Autodesk Inventor part; units mm, degrees
ref_plane "YZ Plane" through (0, 0, 0) normal (1, 0, 0) x (0, 1, 0)
ref_plane "XZ Plane" through (0, 0, 0) normal (0, 1, 0) x (-1, 0, 0)
ref_plane "XY Plane" through (0, 0, 0) normal (0, 0, 1) x (1, 0, 0)
sketch "Sketch1" plane through (0, 0, 0) normal (1, 0, 0) x (0, 1, 0)
  circle A0 centre (0, 0) radius 20
  line L0 (8.5, 8.5) -> (-16.9, 8.5)
  line L1 (8.5, 8.5) -> (8.5, -16.9)
  line L2 (0, 0) -> (0, 20)
  line L3 (0, 20) -> (-60.9241, 20)
  line L4 (-60.9241, 20) -> (-60.9241, 18.5)
  line L5 (-60.9241, 18.5) -> (0, 18.5)
  line L6 (0, 18.5) -> (0, 20)
  line L7 (0, 0) -> (14.1421, 14.1421)
  line L8 (0, 0) -> (20, 0)
  line L9 (-16.9, 8.5) -> (-16.9, 18.5)
  line L10 (-16.9, 8.5) -> (-22.9, 14.5)
  line L11 (-22.9, 14.5) -> (-22.9, 18.5)
  line L12 (12.3744, 12.3744) -> (12.1502, 13.2109)
  line L13 (11.3137, 13.435) -> (9.2071, 11.3284)
  line L14 (9.4313, 10.4919) -> (10.2678, 10.2678)
  line L15 (8.5, 8.5) -> (8.5, -16.9)
  line L16 (20, 0) -> (20, -60.9241)
  line L17 (20, -60.9241) -> (18.5, -60.9241)
  line L18 (18.5, -60.9241) -> (18.5, 0)
  line L19 (8.5, -16.9) -> (18.5, -16.9)
  line L20 (8.5, -16.9) -> (14.5, -22.9)
  line L21 (14.5, -22.9) -> (18.5, -22.9)
  arc A1 (9.2071, 11.3284) -> (9.4313, 10.4919) centre (9.5607, 10.9749) ccw
  arc A2 (12.1502, 13.2109) -> (11.3137, 13.435) centre (11.6673, 13.0815) ccw
  line L22 (10.4311, 10.4311) -> (9.483, 10.6851)
  arc A3 (9.3485, 11.187) -> (9.483, 10.6851) centre (9.5607, 10.9749) ccw
  line L23 (9.3485, 11.187) -> (11.4551, 13.2936)
  arc A4 (11.957, 13.1591) -> (11.4551, 13.2936) centre (11.6673, 13.0815) ccw
  line L24 (11.957, 13.1591) -> (12.2111, 12.2111)
  point P0 (0, 8.5)
  point P1 (-17.7041, 9.3041)
  point P2 (-16.9, 10.6953)
  dimension "d0" = 40
  dimension "d1" = 25.4
  dimension "d2" = 1.5
  dimension "d4" = 45
  dimension "d6" = 45
  dimension "d7" = 4
  dimension "d8" = 10
  dimension "d10" = 2.5
  dimension "d11" = 2.5
  dimension "d12" = 60
  dimension "d13" = 1.5
  dimension "d15" = 0.5
  dimension "d16" = 0.2
extrude "Extrusion1" add sketch "Sketch1" along normal blind 216 contours L7 L12 A2 L13 A1 L14 L0 L2 A0 | L5 L2 L0 L9 A0 | A0 L9 L5 | L9 L10 A0 | A0 L10 L11 L5 L9
sketch "Sketch2" plane through (0, -22.9, 18.5) normal (0, 0, 1) x (1, 0, 0)
  line L0 (0, 22.9) -> (0, 0)
  line L1 (0, 0) -> (216, 0)
  line L2 (216, 22.9) -> (216, 0)
  line L3 (0, 22.9) -> (216, 22.9)
  line L4 (28.3257, 13.1) -> (26.6514, 16)
  line L5 (26.6514, 16) -> (28.3257, 18.9)
  line L6 (28.3257, 18.9) -> (31.6743, 18.9)
  line L7 (31.6743, 18.9) -> (33.3486, 16)
  line L8 (33.3486, 16) -> (31.6743, 13.1)
  line L9 (31.6743, 13.1) -> (28.3257, 13.1)
  line L10 (0, 6) -> (216, 6)
  circle A0 centre (30, 16) radius 1.65
  dimension "d20" = 10
  dimension "d21" = 5.8
  dimension "d22" = 30
  dimension "d25" = 3.3
extrude "Extrusion2" cut sketch "Sketch2" against normal blind 6 contours L4 L5 L6 L7 L8 L9 | A0
extrude "Extrusion3" cut sketch "Sketch2" against normal through all contours A0
sketch "Sketch3" plane through (0, -22.9, 18.5) normal (0, 0, 1) x (1, 0, 0)
  line L0 (0, 37.0421) -> (216, 37.0421)
  line L1 (0, 0) -> (216, 0)
  line L2 (0, 22.9) -> (0, 0)
  line L3 (0, 22.9) -> (0, 37.0421)
  line L4 (2.4384, 37.0421) -> (17.8575, 0)
  line L5 (0, 0) -> (216, 0)
  line L6 (2.4384, 37.0421) -> (0, 42.9)
  point P0 (17.8575, 0)
  dimension "d28" = 112.6
extrude "Extrusion4" cut sketch "Sketch3" along normal through all both and the other way through all
pattern_linear "Rectangular Pattern1" count 2 spacing 150 along (1, 0, 0) of "Extrusion3", "Extrusion2"
properties part number "ESQUINA_REDONDEADA_R20" material "Steel, Mild, Welded"
The listing builds one solid part. Answer for the finished solid, in the listing's coordinates (mm). A direction names the side the tool comes from. Coordinates: 2 decimals unless noted, no trailing zeros. Loops run counter-clockwise (first coordinate to the right, second up) from the corner with the lowest first, then second, coordinate; pieces in that order, holes last. Notation, with made-up numbers: M 68.25,34.25 L 72.25,34.25 A21 ccw 72.25,38.25 Z; hole C 10.5,38 d9. An arc over 180 degrees is marked long. Answer as a JSON object with one key per item and string values. Group by question number.
Item 1: Section A-A (x = 112.5) is taken. Write down the section's boundary in (y, z) (3 decimals), and give its area (3 significant figures).
Item 2: Determine the mould class of faces 1 (the face through (109, -4, 8.5)), 2 (the face through (107.7, 7.6, 18.5)), 3 (the face through (31.4, -5.6, 12.5)) for opening direction Y: +Y half, -Y half, draft (parallel to the pull), parting line (faces both ways), or undercut.
Item 3: Which of the six approach directions +Z, -Z, +X, -X, +Y, -Y give full straight-line access (tool end or side, diameter ignored) to faces 4 (the face through (180, -4, 16)), 5 (the face through (111, -12, 18.5)), 6 (the face through (181.574, -6.404, 10.528))?
Item 4: Each of these flat-tipped pins is pushed along its axis until it touches: P1, Ø4, axis at x = 93.5, z = 11, coming from the -Y side; P2, Ø1, axis at x = 180, z = 15, coming from the +Y side (3 decimals); P3, Ø2, axis at x = 30, y = -6.9, coming from the +Z side; P4, Ø4, axis at x = 76, z = 12.5, coming from the +Y side. Where does it stop, or does it pass through?
Item 5: Consider L1, parallel to Z at x = 85.5, y = -7.5; L2, parallel to Y at x = 30, z = 9.75; L3, parallel to X at y = -17, z = 12.75. Determine where each line is inside the solid, lowest interval first.
Item 6: Section B-B (y = -13.5) is taken. Write down the section's boundary in (x, z).
Solved:
{
 "1": {"outline": "M -22.9,14.5 L -16.9,8.5 L 8.5,8.5 L 10.268,10.268 L 9.431,10.492 A0.5 cw 9.207,11.328 L 11.314,13.435 A0.5 cw 12.15,13.211 L 12.374,12.374 L 14.142,14.142 A20 ccw 0,20 L 0,18.5 L -22.9,18.5 Z", "area": "327 mm2"},
 "2": {"face 1": "draft", "face 2": "+Y half", "face 3": "undercut"},
 "3": {"face 4": "+Z", "face 5": "+Z, +X, -X, -Y", "face 6": "+Z, -Z"},
 "4": {"P1": "stops at y = -21.4", "P2": "stops at y = 13.775", "P3": "passes through", "P4": "stops at y = 14.14"},
 "5": {"L1": "z = 8.5 to 18.5", "L2": "y = -18.15 to -8.55, -5.25 to 9.75", "L3": "x = 15.4 to 216"},
 "6": {"outline": "M 13.94,8.5 L 216,8.5 L 216,18.5 L 13.94,18.5 Z"}
}
